Job drawing, mm, ordinate dimensions from the low corner. One solid piece. A direction names the side the tool comes from. Give positions to 0.01 mm unless a question says otherwise; leave off trailing zeros. Order: outer loops, then holes, each group sorted by start corner. A loop starts at its lowest first (then second) coordinate and runs counter-clockwise, first axis right, second up. Notation, with made-up numbers: M 6.5,25 L 60.5,25 A18 cw 60.5,43 Z; hole C 24.5,43 d2. An arc over 180 degrees is marked long. Use CSV: the item, a comma, the result in double quotes. Start each with the question number.
Item 1: Two-plate mould, pull along Y, no slides. Class the marked faces 1, 2 and 3: pulls with the +Y half, pulls with the -Y half, needs draft (parallel to the pull), parting line crosses it, or undercut.
Item 2: Wall check: line 1 along Z through (x, y) = (24.5, 18); line 2 along X through (y, z) = (16, 15.25). Give the ranges that are in metal, low to high.
Item 3: Which spindle directions (+Z, -Z, +X, -X, +Y, -Y) get a long thin tool onto all of the face, cutting with end or side? Do the marked faces 4 and 5. Say none if no direction does.
Item 4: Band-saw the part on B-B on x = 8. Write the cut outline in (y, z), plus the area to 3 significant figures.
Item 5: Band-saw the part on A-A on y = 11.5. Write the cut outline in (x, z) (1 decimal).
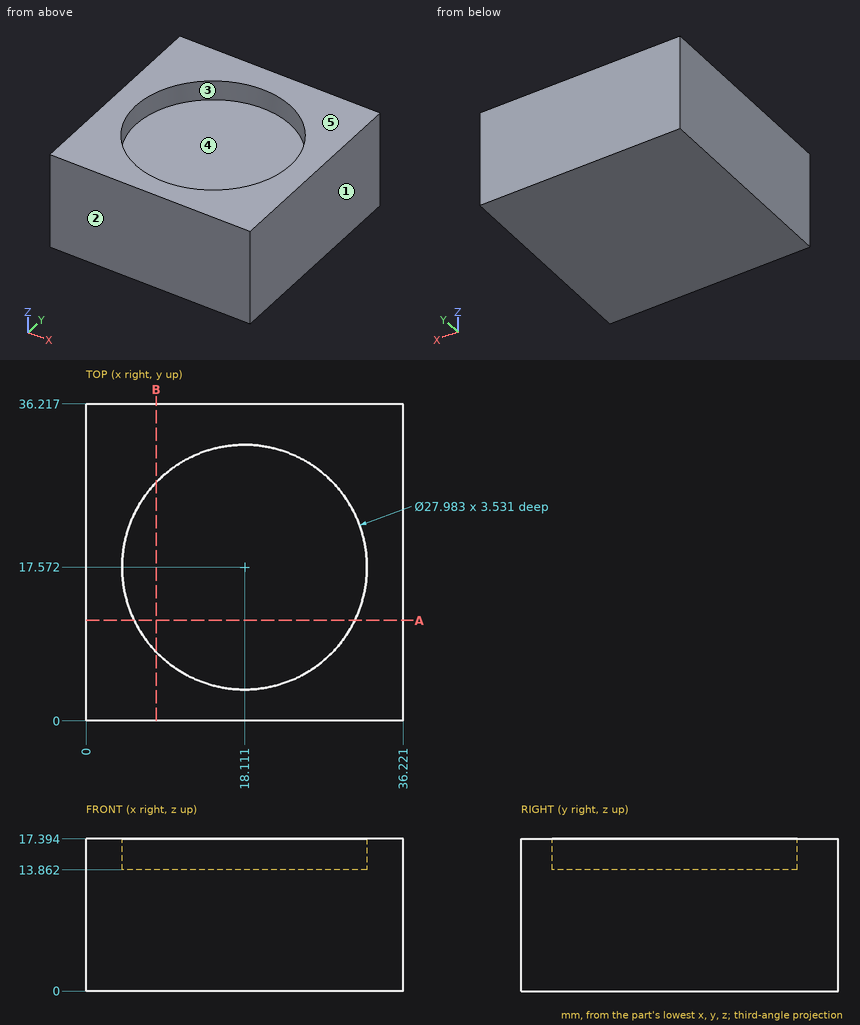
Model answer:
1,face 1,"needs draft"
1,face 2,"pulls with the -Y half"
1,face 3,"undercut"
2,line 1,"z = 0 to 13.86"
2,line 2,"x = 0 to 4.21, 32.01 to 36.22"
3,face 4,"+Z"
3,face 5,"+Z, +X, -X, +Y, -Y"
4,outline,"M 0,0 L 36.22,0 L 36.22,17.39 L 27.24,17.39 L 27.24,13.86 L 7.9,13.86 L 7.9,17.39 L 0,17.39 Z"
4,area,"562 mm^2"
5,outline,"M 0,0 L 36.2,0 L 36.2,17.4 L 30.7,17.4 L 30.7,13.9 L 5.5,13.9 L 5.5,17.4 L 0,17.4 Z"
